Can you work these out from the model? Positions are in its coordinate system, mm. A direction names the side the tool comes from. Round coordinates to 2 decimals unless told otherwise and drop trailing zeros. Write each loop counter-clockwise with the first axis right and the second up, starting at its lowest first coordinate (ties: lowest second). Pieces come first, ordered by that corner, then holes. Notation, with made-up numbers: M 89.25,10.5 L 102.25,10.5 A29 ccw 102.25,47.5 Z; hole C 32.5,38 d1. An arc over 180 degrees is marked long. Answer in a Markdown table with one row per item. Add a question column.
(1) Suppose I cut it at A-A, the plane y = 0. Count the separate pieces of the cut face and the enclosed holes in it, then the cut area to 3 significant figures.
(2) Suppose I cut it at D-D, the plane x = 16.57. Write out the boundary of the cut face in (y, z).
(3) For faces 1 (the face through (2.588, 11.654, -1.961)), 2 (the face through (1.9, 14.44, 0.23)), 3 (the face through (-6.466, 2.681, -3.714)), which set-ups out of +Z, -Z, +X, -X, +Y, -Y let a thin tool reach every point of the face, with its end or its side?
(4) Suppose I cut it at C-C, the plane z = 7.25. Write out the boundary of the cut face in (x, y), then the cut area to 3 significant figures.
(5) If I drill on probe 1 along Z at (x, y) = (11, -12.5); probe 2 along Z at (x, y) = (-6.5, -11); probe 3 along Y at (x, z) = (3.5, -2), over which ranges is the centre line in solid material (lowest first)?
(6) If we mould it in two halves opening along Y, with no side actions, what happens to faces 4 (the face through (-5.1, 5.1, -2.7)), 5 (the face through (2.55, -19.45, 7.27)), 6 (the face through (3.4, 6.3, -4.7))? For each: released by +Y, released by -Y, zero draft, split by the parting line, or undercut.
(7) I'm going to push flat-ended pins straight in: pin 1 (6 mm diameter, centred on x = -11, z = 0.5, fed in from -Y); pin 2 (8 mm diameter, centred on x = -5.5, y = 4, fed in from +Z); pin 3 (8 mm diameter, centred on x = 1.5, z = -3, fed in from -Y) (3 decimals). Where does each tip first touch, or does it pass through?
(8) Suppose I cut it at B-B, the plane x = 0. Write out the boundary of the cut face in (y, z) (3 decimals), then the cut area to 3 significant figures.
from build123d import *

# Parameters (mm, degrees)
SKETCH1_W          = 12.617819502
SKETCH1_H          = 2
SKETCH1_W_2        = 6.5532
SKETCH1_H_2        = 9.89
SKETCH2_R          = 26.652766262
SKETCH2_R_2        = 14.565
CUT_EXTRUDE1_DEPTH = 10
SKETCH4_R          = 1.0922
CUT_EXTRUDE2_DEPTH = 30.490976315
CHAMFER1_SIZE      = 0.5


with BuildPart() as part:
    # Sketch1 → Revolve1 (revolve)
    with BuildSketch(Plane(origin=(0, 0, 0), x_dir=(1, 0, 0), z_dir=(0, 1, 0))):
        with Locations((-13.308909751, 3.700473465)):
            Rectangle(SKETCH1_W, SKETCH1_H)
        Polygon((-11.938, 2.700473465), (-19.617819502, 2.700473465), (-19.617819502, 0.700473465), (-13.064619502, 0.700473465), (-11.938, 0.700473465), align=None)
        with Locations((-16.341219502, -4.244526535)):
            Rectangle(SKETCH1_W_2, SKETCH1_H_2)
    revolve(axis=Axis((0, 0, -25.411285606), (0, 0, 1)))

    # Sketch2 → Cut-Extrude1 (cut)
    with BuildSketch(Plane(origin=(0, 0, -4.700473465), x_dir=(-1, 0, 0), z_dir=(0, 0, -1))):
        Circle(SKETCH2_R)
        Circle(SKETCH2_R_2, mode=Mode.SUBTRACT)
    extrude(amount=-CUT_EXTRUDE1_DEPTH, mode=Mode.SUBTRACT)

    # Sketch4 → Cut-Extrude2 (cut, through all)
    with BuildSketch(Plane(origin=(0, 0, 5.299526535), x_dir=(-1, 0, 0), z_dir=(0, 0, -1))):
        with Locations((16.57, 0)):
            Circle(SKETCH4_R)
        with Locations(Location((-16.57, 0, 0), (0, 0, 180))):
            Circle(SKETCH4_R)
    extrude(amount=-CUT_EXTRUDE2_DEPTH, mode=Mode.SUBTRACT)

    # Chamfer1
    chamfer1_edges = [part.edges().sort_by_distance(p)[0] for p in [
        (11.938, 0, -0.700473465),
    ]]
    chamfer(chamfer1_edges, length=CHAMFER1_SIZE)


solid = part.part
Calculated:
| question | item | result |
|---|---|---|
| 1 | separate pieces | 4 |
| 1 | enclosed holes | 0 |
| 1 | area | 92.5 mm² |
| 2 | outline | M -10.5,5.3 L -1.09,5.3 L -1.09,9.19 L -10.5,9.19 Z; M 1.09,5.3 L 10.5,5.3 L 10.5,9.19 L 1.09,9.19 Z |
| 3 | face 1 | +Z |
| 3 | face 2 | -Z |
| 3 | face 3 | +Z, -Z |
| 4 | outline | C 0,0 d39.24; hole C -16.57,0 d2.18; hole C 0,0 d26.13; hole C 16.57,0 d2.18 |
| 4 | area | 665 mm² |
| 5 | probe 1 | 5.3 to 9.19 |
| 5 | probe 2 | -4.7 to -0.7 |
| 5 | probe 3 | -14.14 to -11.41, 11.41 to 14.14 |
| 6 | face 4 | undercut |
| 6 | face 5 | split by the parting line |
| 6 | face 6 | zero draft |
| 7 | pin 1 | y = -12.17 |
| 7 | pin 2 | z = -2.7 |
| 7 | pin 3 | y = -14.565 |
| 8 | outline | M -19.618,5.3 L -14.565,5.3 L -14.565,-4.7 L -7,-4.7 L -7,-2.7 L -11.938,-2.7 L -11.938,-1.2 L -12.438,-0.7 L -13.065,-0.7 L -13.065,9.19 L -19.618,9.19 Z; M 7,-4.7 L 14.565,-4.7 L 14.565,5.3 L 19.618,5.3 L 19.618,9.19 L 13.065,9.19 L 13.065,-0.7 L 12.438,-0.7 L 11.938,-1.2 L 11.938,-2.7 L 7,-2.7 Z |
| 8 | area | 110 mm² |
